Verification items for the finished model (mm, model axes). A direction names the side the tool comes from. Round coordinates to 2 decimals unless told otherwise and drop trailing zeros. Write each loop counter-clockwise with the first axis right and the second up, starting at its lowest first coordinate (ties: lowest second). Pieces come first, ordered by that corner, then holes. Notation, with made-up numbers: M 29.5,12 L 33.5,12 A31 cw 33.5,42 Z; hole C 71.5,37 d10. An arc over 180 degrees is marked long. One line per item, written item: value. Start each with the question number.
from build123d import *

# Parameters (mm, degrees)
SKETCH1_W           = 30.48
SKETCH1_H           = 30.48
BOSS_EXTRUDE1_DEPTH = 5.08
FILLET1_R           = 2.54
SKETCH2_R           = 3.81
BOSS_EXTRUDE2_DEPTH = 97.79
SKETCH3_R           = 2.54
CUT_EXTRUDE1_DEPTH  = 101.6


with BuildPart() as part:
    # Sketch1 → Boss-Extrude1 (new body)
    with BuildSketch(Plane(origin=(0, 0, 0), x_dir=(1, 0, 0), z_dir=(0, 1, 0))):
        Rectangle(SKETCH1_W, SKETCH1_H)
    extrude(amount=BOSS_EXTRUDE1_DEPTH)

    # Fillet1
    fillet1_edges = [part.edges().sort_by_distance(p)[0] for p in [
        (-15.24, 5.08, 0),
        (0, 5.08, 15.24),
        (15.24, 5.08, 0),
        (0, 5.08, -15.24),
    ]]
    fillet(fillet1_edges, radius=FILLET1_R)

    # Sketch2 → Boss-Extrude2 (add)
    with BuildSketch(Plane.XZ):
        Circle(SKETCH2_R)
    extrude(amount=BOSS_EXTRUDE2_DEPTH)

    # Sketch3 → Cut-Extrude1 (cut)
    with BuildSketch(Plane(origin=(0, 5.08, 0), x_dir=(1, 0, 0), z_dir=(0, 1, 0))):
        Circle(SKETCH3_R)
    extrude(amount=-CUT_EXTRUDE1_DEPTH, mode=Mode.SUBTRACT)


solid = part.part
1) Thickness scan on line 1 (Z direction, x = 0, y = -24); line 2 (Y direction, x = 12, z = 9); line 3 (X direction, y = -10.5, z = -1). Record the ranges inside material, lowest first.
2) Cross-section at D-D (z = 5.5). Record the boundary of the cut face in (x, y), then the cut area to 3 significant figures.
3) Cross-section at B-B (z = 0). Record the boundary of the cut face in (x, y), then the cut area to 3 significant figures.
4) Mould release check, pull along X, two halves, no side actions. Record for faces 3 (the flat face through (0, -97.79, 0)), 4 (the flat face through (0, -96.52, 0)), 5 (the cylindrical face through (-0.83, -48.21, -3.72)), 6 (the cylindrical face through (-0.33, -45.01, -2.52)): pulls with the +X half, pulls with the -X half, needs draft (parallel to the pull), parting line crosses it, or undercut.
5) Cross-section at C-C (y = -29.5). Record the boundary of the cut face in (x, z).
6) Access from +Z, -Z, +X, -X, +Y, -Y to the whole of each face (thin tool, end or side, straight path). Record for faces 1 (the flat face through (15.24, 1, 0)), 2 (the flat face through (3, 0, -4)).
7) Gauge pin test, flat ends, axial feed: pin 1 Ø5 at (y, z) = (-81, -5) entering from -X; pin 2 Ø1 at (x, z) = (-6.5, 3.5) entering from -Y; pin 3 Ø4 at (x, y) = (7, -47.5) entering from -Z; pin 4 Ø1 at (x, y) = (3, -10.5) entering from -Z. Record the tip position at first contact, or that the pin passes through.
8) Cross-section at A-A (x = 0). Record the boundary of the cut face in (y, z), then the cut area to 3 significant figures.
Results below:
1. line 1: z = -3.81 to -2.54, 2.54 to 3.81
1. line 2: y = 0 to 5.08
1. line 3: x = -3.68 to -2.33, 2.33 to 3.68
2. outline: M -15.24,0 L 15.24,0 L 15.24,2.54 A2.54 ccw 12.7,5.08 L -12.7,5.08 A2.54 ccw -15.24,2.54 Z
2. area: 152 mm²
3. outline: M -15.24,0 L -3.81,0 L -3.81,-97.79 L 3.81,-97.79 L 3.81,0 L 15.24,0 L 15.24,2.54 A2.54 ccw 12.7,5.08 L 2.54,5.08 L 2.54,-96.52 L -2.54,-96.52 L -2.54,5.08 L -12.7,5.08 A2.54 ccw -15.24,2.54 Z
3. area: 381 mm²
4. face 3: needs draft
4. face 4: undercut
4. face 5: parting line crosses it
4. face 6: undercut
5. outline: C 0,0 d7.62; hole C 0,0 d5.08
6. face 1: +Z, -Z, +X, +Y, -Y
6. face 2: -Y
7. pin 1: stops at x = -2.88
7. pin 2: stops at y = 0
7. pin 3: passes through
7. pin 4: stops at z = -2.88
8. outline: M -97.79,-3.81 L 0,-3.81 L 0,-15.24 L 2.54,-15.24 A2.54 ccw 5.08,-12.7 L 5.08,-2.54 L -96.52,-2.54 L -96.52,2.54 L 5.08,2.54 L 5.08,12.7 A2.54 ccw 2.54,15.24 L 0,15.24 L 0,3.81 L -97.79,3.81 Z
8. area: 381 mm²
